Geometry check sheet. Reference: the model listing, model coordinates, mm. Face numbers are marked on the shaded views. A direction names the side the tool comes from. Coordinates: 2 decimals unless noted, no trailing zeros. Write each loop counter-clockwise with the first axis right and the second up, starting at its lowest first coordinate (ties: lowest second). Pieces come first, ordered by that corner, then holes. Notation, with made-up numbers: M -3.75,72 L 39.25,72 A34 cw 39.25,111 Z; hole C 73.5,16.5 d10. An arc over 180 degrees is marked long. Put each result on its own line as item: value. Start each with the question number.
1) Set-up check for the marked faces 1 and 2: record each of +Z, -Z, +X, -X, +Y, -Y from which the full face is reachable in a straight line by a thin tool's end or side.
2) Cross-section at D-D on x = 11. Record the cut outline in (y, z), plus the area to 3 significant figures.
3) Gauge pin test, flat ends, axial feed: pin 1 (1.5 mm diameter, centred on x = 4, z = -3, fed in from +Y); pin 2 (0.8 mm diameter, centred on x = 1, y = 0.5, fed in from +Z); pin 3 (2.5 mm diameter, centred on x = 5.16, y = 14.36, fed in from +Z); pin 4 (6 mm diameter, centred on x = 10, z = -2.5, fed in from +Y). Record the tip position at first contact, or that the pin passes through.
4) Cross-section at B-B on x = 4.75. Record the cut outline in (y, z), plus the area to 3 significant figures.
5) Cross-section at A-A on x = 15. Record the cut outline in (y, z).
6) Scan lines: line 1 along Y through (x, z) = (4, -11.5); line 2 along Z through (x, y) = (11.75, 3); line 3 along Y through (x, z) = (4, -0.75). Record each from-to range of solid material in increasing order.
7) Cross-section at C-C on y = 14. Record the cut outline in (x, z).
Autodesk Inventor part; units mm, degrees
ref_plane "c2_XY" through (0, 0, 0) normal (1, 0, 0) x (0, 0, -1)
ref_plane "c2_YZ" through (0, 0, 0) normal (0, 0, -1) x (0, 1, 0)
ref_plane "c2_ZX" through (0, 0, 0) normal (0, 1, 0) x (1, 0, 0)
sketch "Sketch_1" plane through (0, 0, 0) normal (1, 0, 0) x (0, 1, 0)
  line L0 (19.558, 0) -> (1.27, 0)
  arc A0 (1.27, 0) -> (0, -1.27) centre (1.27, -1.27) ccw
  line L1 (0, -1.27) -> (0, -12.954)
  line L2 (0, -12.954) -> (1.5189, -12.954)
  line L3 (1.5189, -12.954) -> (1.5189, -2.7889)
  arc A1 (2.7889, -1.5189) -> (1.5189, -2.7889) centre (2.7889, -2.7889) ccw
  line L4 (2.7889, -1.5189) -> (19.558, -1.5189)
  line L5 (19.558, -1.5189) -> (19.558, 0)
extrude "Extrusion1" add sketch "Sketch_1" along normal blind 19.05
sketch "Sketch_2" plane through (0, 0, 0) normal (0, 0, 1) x (1, 0, 0)
  line L0 (-19.05, -19.558) -> (28.575, -19.558)
  line L1 (28.575, -19.558) -> (28.575, 29.337)
  line L2 (28.575, 29.337) -> (-19.05, 29.337)
  line L3 (-19.05, 29.337) -> (-19.05, -19.558)
  line L4 (0, 0) -> (19.05, 0)
  line L5 (19.05, 0) -> (19.05, 3.175)
  line L6 (19.05, 3.175) -> (9.4129, 17.2734)
  arc A0 (9.4129, 17.2734) -> (0, 14.3637) centre (5.1562, 14.3637) ccw
  line L7 (0, 14.3637) -> (0, 0)
extrude "Extrusion2" cut sketch "Sketch_2" against normal blind 12.954
sketch "Sketch3" plane through (0, 1.27, 0) normal (0, 0, 1) x (1, 0, 0)
  point P0 (5.1562, 13.0937)
hole "Hole1" at (5.1562, 14.3637, 0) direction (0, 0, -1) diameter 4.0259 depth 1.5189
sketch "Sketch4" plane through (0, 0, -12.954) normal (0, -1, 0) x (1, 0, 0)
  point P0 (3.175, 5.7531)
hole "Hole2" at (3.175, 0, -7.2009) direction (0, 1, 0) diameter 4.826 depth 1.5189
sketch "Sketch5" plane through (0, 0, -12.954) normal (0, -1, 0) x (1, 0, 0)
  point P0 (15.875, 5.7531)
hole "Hole3" at (15.875, 0, -7.2009) direction (0, 1, 0) diameter 4.826 depth 1.5189
sketch "Sketch_6" plane through (0, 0, 0) normal (0, 1, 0) x (-1, 0, 0)
  line L0 (0, -9.6139) -> (0, -4.7879)
  line L1 (0, -4.7879) -> (-3.175, -4.7879)
  line L2 (-3.175, -4.7879) -> (-3.175, -9.6139)
  line L3 (-3.175, -9.6139) -> (0, -9.6139)
sketch "Sketch_7" plane through (0, 0, 0) normal (0, 1, 0) x (-1, 0, 0)
  line L0 (-15.875, -9.6139) -> (-15.875, -4.7879)
  line L1 (-15.875, -4.7879) -> (-19.05, -4.7879)
  line L2 (-19.05, -4.7879) -> (-19.05, -9.6139)
  line L3 (-19.05, -9.6139) -> (-15.875, -9.6139)
extrude "Extrusion3" cut sketch "Sketch_6" along normal blind 1.5189
extrude "Extrusion4" cut sketch "Sketch_7" along normal blind 1.5189
sketch "Sketch_8" plane through (0, 0, 0) normal (0, 1, 0) x (-1, 0, 0)
  line L0 (0, -19.431) -> (0, -11.684)
  arc A0 (-1.27, -12.954) -> (0, -11.684) centre (-1.27, -11.684) ccw
  line L1 (-1.27, -12.954) -> (-17.78, -12.954)
  arc A1 (-19.05, -11.684) -> (-17.78, -12.954) centre (-17.78, -11.684) ccw
  line L2 (-19.05, -11.684) -> (-19.05, -19.431)
  line L3 (-19.05, -19.431) -> (0, -19.431)
extrude "Extrusion5" cut sketch "Sketch_8" along normal blind 1.5189
ref_plane "c2_XY" through (0, 0, 0) normal (1, 0, 0) x (0, 0, -1)
ref_plane "c2_YZ" through (0, 0, 0) normal (0, 0, -1) x (0, 1, 0)
ref_plane "c2_ZX" through (0, 0, 0) normal (0, 1, 0) x (1, 0, 0)
ref_plane "k2_XY" through (0, 0, -12.954) normal (1, 0, 0) x (0, 0, -1)
ref_plane "k2_YZ" through (0, 0, -12.954) normal (0, 0, -1) x (0, 1, 0)
ref_plane "k2_ZX" through (0, 0, -12.954) normal (0, 1, 0) x (1, 0, 0)
ref_plane "to_dummy_R_XY" through (0, 0, 0) normal (0, 0, 1) x (1, 0, 0)
ref_plane "to_dummy_R_YZ" through (0, 0, 0) normal (1, 0, 0) x (0, 1, 0)
ref_plane "to_dummy_R_ZX" through (0, 0, 0) normal (0, 1, 0) x (0, 0, 1)
ref_plane "to_pin_R_XY" through (5.1562, 14.3637, 0) normal (0, 0, 1) x (1, 0, 0)
ref_plane "to_pin_R_YZ" through (5.1562, 14.3637, 0) normal (1, 0, 0) x (0, 1, 0)
ref_plane "to_pin_R_ZX" through (5.1562, 14.3637, 0) normal (0, 1, 0) x (0, 0, 1)
properties part number "D-782_pin" material "Steel"
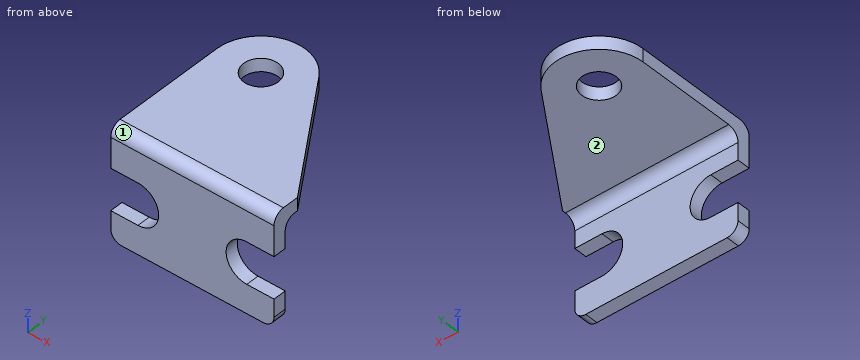
Answer key:
1. face 1: +Z, +X, -X, -Y
1. face 2: -Z, +X, -X, +Y
2. outline: M 0,-12.95 L 1.52,-12.95 L 1.52,-2.79 A1.27 cw 2.79,-1.52 L 14.95,-1.52 L 14.95,0 L 1.27,0 A1.27 ccw 0,-1.27 Z
2. area: 40.1 mm²
3. pin 1: stops at y = 1.64
3. pin 2: stops at z = -0.06
3. pin 3: passes through
3. pin 4: stops at y = 19.11
4. outline: M 0,-12.95 L 1.52,-12.95 L 1.52,-9.03 L 0,-9.03 Z; M 0,-5.37 L 1.52,-5.37 L 1.52,-2.79 A1.27 cw 2.79,-1.52 L 12.39,-1.52 L 12.39,0 L 1.27,0 A1.27 ccw 0,-1.27 Z; M 16.34,-1.52 L 19.5,-1.52 L 19.5,0 L 16.34,0 Z
4. area: 35.5 mm²
5. outline: M 0,-12.95 L 1.52,-12.95 L 1.52,-9.45 L 0,-9.45 Z; M 0,-4.95 L 1.52,-4.95 L 1.52,-2.79 A1.27 cw 2.79,-1.52 L 9.1,-1.52 L 9.1,0 L 1.27,0 A1.27 ccw 0,-1.27 Z
6. line 1: y = 0 to 1.52
6. line 2: z = -1.52 to 0
6. line 3: y = 0.11 to 12.72, 16.01 to 19.39
7. outline: M 0,-1.52 L 3.18,-1.52 L 3.18,0 L 0,0 Z; M 7.14,-1.52 L 11.65,-1.52 L 11.65,0 L 7.14,0 Z
